```python
from build123d import *

# Parameters (mm, degrees)
P_IDAT_VYSUNUT_M1_DEPTH  = 8
ODEBRAT_VYSUNUT_M1_DEPTH = 153.557332159
SKICA5_W                 = 16
SKICA5_H                 = 8
P_IDAT_VYSUNUT_M2_DEPTH  = 8
ODEBRAT_VYSUNUT_M4_DEPTH = 153.557332159
SKICA4_W                 = 2.4
SKICA4_H                 = 2.4
ODEBRAT_VYSUNUT_M2_DEPTH = 4.4
SKICA9_R                 = 2.2
ODEBRAT_VYSUNUT_M5_DEPTH = 9.4


with BuildPart() as part:
    # Skica2 → Přidat vysunutím1 (new body)
    with BuildSketch(Plane(origin=(0, 0, 0), x_dir=(1, 0, 0), z_dir=(0, 1, 0))):
        Polygon((0, 0), (0, -27.47211487), (-149.85, 0.000769495), (-108.259653873, 0.000769495), (-72.85, -6.491091207), (-72.85, 0), (-65.55, 0), (-65.55, -7.829443265), (-7.3, -18.508759343), (-7.3, 0), align=None)
    extrude(amount=P_IDAT_VYSUNUT_M1_DEPTH)

    # Skica3 → Odebrat vysunutím1 (cut, through all)
    with BuildSketch(Plane(origin=(0, 8, 0), x_dir=(1, 0, 0), z_dir=(0, 1, 0))):
        Polygon((0, -20), (-1, -20), (-3.2, -18), (-3.2, -24.4), (-1, -22.4), (0, -22.4), align=None)
    extrude(amount=-ODEBRAT_VYSUNUT_M1_DEPTH, mode=Mode.SUBTRACT)

    # Skica5 → Přidat vysunutím2 (add)
    with BuildSketch(Plane(origin=(0, 8, 0), x_dir=(1, 0, 0), z_dir=(0, 1, 0))):
        with Locations((-8, -4)):
            Rectangle(SKICA5_W, SKICA5_H)
    extrude(amount=-P_IDAT_VYSUNUT_M2_DEPTH)

    # Skica7 → Odebrat vysunutím4 (cut, through all)
    with BuildSketch(Plane.XZ):
        Polygon((-7.3, 8), (-16, 8), (-16, 0), align=None)
    extrude(amount=-ODEBRAT_VYSUNUT_M4_DEPTH, mode=Mode.SUBTRACT)

    # Skica4 → Odebrat vysunutím2 (cut)
    with BuildSketch(Plane(origin=(0, 0, 0), x_dir=(0, 0, -1), z_dir=(1, 0, 0))):
        with Locations((-13.2, 4)):
            Rectangle(SKICA4_W, SKICA4_H)
    extrude(amount=-ODEBRAT_VYSUNUT_M2_DEPTH, mode=Mode.SUBTRACT)

    # Skica9 → Odebrat vysunutím5 (cut)
    with BuildSketch(Plane(origin=(0, 0, 0), x_dir=(-1, 0, 0), z_dir=(0, 0, -1))):
        with Locations((3.65, 4)):
            Circle(SKICA9_R)
        with Locations((69.2, 4)):
            Circle(SKICA9_R)
    extrude(amount=-ODEBRAT_VYSUNUT_M5_DEPTH, mode=Mode.SUBTRACT)


solid = part.part
```
Here's how the part is built. I have some questions about the finished solid (model axes, mm). A direction names the side the tool comes from. Give positions to 0.01 mm unless a question says otherwise; leave off trailing zeros. Order: outer loops, then holes, each group sorted by start corner. A loop starts at its lowest first (then second) coordinate and runs counter-clockwise, first axis right, second up. Notation, with made-up numbers: (21, 74.25) -> (43, 74.25) arc R21 ccw to (43, 85.25) -> close; hole circle Ø8 at (57.25, 56.25). An arc over 180 degrees is marked (long way). Use CSV: the item, a comma, the result in double quotes. Start each with the question number.
Item 1: Suppose I cut it at D-D (x = -69.2). List the corners of the cut face in (y, z) for me.
Item 2: If I drill on probe 1 along Y at (x, z) = (-69.2, 5.5); probe 2 along Z at (x, y) = (-13.5, 7); probe 3 along Z at (x, y) = (-10, 0.75), over which ranges is the centre line in solid material (lowest first)? Write a range as [from, to].
Item 3: Thinking about a two-plate mould opening in Z: for faces 1 (the flat face through (-73.876, 3.944, 13.928)), 2 (the flat face through (-72.85, 4, 3)), 3 (the flat face through (-2, 5.2, 13)), which applies, pulls with the +Z half, pulls with the -Z half, needs draft (parallel to the pull), parting line crosses it, or undercut?
Item 4: On a 3-axis mill with a long thin cutter (end or side, diameter ignored), from which of +Z, -Z, +X, -X, +Y, -Y can I reach the whole of each face in a straight line? I mean faces 4 (the flat face through (-11.711, 3.944, 3.944)), 5 (the flat face through (-2, 4, 14.4)), 6 (the flat face through (-4, 4, 9.4)), 7 (the flat face through (-65.55, 4, 4)). Say none if no direction works.
Item 5: I'm going to push flat-ended pins straight in: P1, Ø4, axis at x = -69.2, y = 4, coming from the -Z side; P2, Ø2, axis at x = -4.5, y = 3, coming from the -Z side; P3, Ø0.5, axis at x = -0.5, y = 6, coming from the +Z side; P4, Ø8, axis at x = -54, z = 4, coming from the +Y side. Where does each tip first touch, or does it pass through?
Item 6: Suppose I cut it at C-C (x = -10). List the corners of the cut face in (y, z) for me, and give its area (3 significant figures).
Item 7: Suppose I cut it at B-B (z = 2.5). List the corners of the cut face in (x, y) for me, and give its area (3 significant figures).
Answer block:
1,outline,"(0, 0) -> (1.8, 0) -> (1.8, 9.4) -> (6.2, 9.4) -> (6.2, 0) -> (8, 0) -> (8, 14.79) -> (0, 14.79) -> close"
2,probe 1,"y = [0, 1.8], [6.2, 8]"
2,probe 2,"z = [0, 2.3], [17.37, 25]"
2,probe 3,"z = [0, 5.52], [18.01, 25.64]"
3,face 1,"pulls with the +Z half"
3,face 2,"needs draft"
3,face 3,"undercut"
4,face 4,"+Y, -Y"
4,face 5,"+X"
4,face 6,"-Z"
4,face 7,"-Z, +Y, -Y"
5,P1,"stops at z = 9.4"
5,P2,"stops at z = 0"
5,P3,"stops at z = 27.43"
5,P4,"passes through"
6,outline,"(0, 0) -> (8, 0) -> (8, 5.52) -> (0, 5.52) -> close; (0, 18.01) -> (8, 18.01) -> (8, 25.64) -> (0, 25.64) -> close"
6,area,"105 mm^2"
7,outline,"(-136.21, 0) -> (-94.62, 0) -> (-94.62, 8) -> (-136.21, 8) -> close; (-72.85, 0) -> (-65.55, 0) -> (-65.55, 8) -> (-72.85, 8) -> close; (-13.28, 0) -> (0, 0) -> (0, 8) -> (-13.28, 8) -> close; hole circle Ø4.4 at (-69.2, 4); hole circle Ø4.4 at (-3.65, 4)"
7,area,"467 mm^2"
